from build123d import *

# Parameters (mm, degrees)
BOSS_EXTRUDE3_DEPTH = 25
SKETCH3_R           = 10
CUT_EXTRUDE1_DEPTH  = 25
SKETCH4_R           = 12.5
CUT_EXTRUDE2_DEPTH  = 15
SKETCH5_R           = 50
BOSS_EXTRUDE5_DEPTH = 75
SKETCH9_R           = 42.5
CUT_EXTRUDE5_DEPTH  = 15
SKETCH10_R          = 37.5
CUT_EXTRUDE6_DEPTH  = 60


with BuildPart() as part:
    # Sketch2 → Boss-Extrude3 (new body)
    with BuildSketch(Plane(origin=(0, 0, 0), x_dir=(1, 0, 0), z_dir=(0, 1, 0))):
        with BuildLine():
            Line((-125, 19.364916731), (-12.5, 48.412291828))
            ThreePointArc((-12.5, 48.412291828), (0, 50), (12.5, 48.412291828))
            Line((12.5, 48.412291828), (125, 19.364916731))
            ThreePointArc((125, 19.364916731), (140, 0), (125, -19.364916731))
            Line((125, -19.364916731), (12.5, -48.412291828))
            ThreePointArc((12.5, -48.412291828), (0, -50), (-12.5, -48.412291828))
            Line((-12.5, -48.412291828), (-125, -19.364916731))
            ThreePointArc((-125, -19.364916731), (-140, 0), (-125, 19.364916731))
        make_face()
    extrude(amount=BOSS_EXTRUDE3_DEPTH)

    # Sketch3 → Cut-Extrude1 (cut)
    with BuildSketch(Plane(origin=(0, 25, 0), x_dir=(1, 0, 0), z_dir=(0, 1, 0))):
        with Locations((-120, 0)):
            Circle(SKETCH3_R)
        with Locations((120, 0)):
            Circle(SKETCH3_R)
    extrude(amount=-CUT_EXTRUDE1_DEPTH, mode=Mode.SUBTRACT)

    # Sketch4 → Cut-Extrude2 (cut)
    with BuildSketch(Plane(origin=(0, 25, 0), x_dir=(1, 0, 0), z_dir=(0, 1, 0))):
        with Locations((-120, 0)):
            Circle(SKETCH4_R)
        with Locations((120, 0)):
            Circle(SKETCH4_R)
    extrude(amount=-CUT_EXTRUDE2_DEPTH, mode=Mode.SUBTRACT)

    # Sketch5 → Boss-Extrude5 (add)
    with BuildSketch(Plane(origin=(0, 0, 0), x_dir=(1, 0, 0), z_dir=(0, 1, 0))):
        Circle(SKETCH5_R)
    extrude(amount=BOSS_EXTRUDE5_DEPTH)

    # Sketch9 → Cut-Extrude5 (cut)
    with BuildSketch(Plane(origin=(0, 75, 0), x_dir=(1, 0, 0), z_dir=(0, 1, 0))):
        Circle(SKETCH9_R)
    extrude(amount=-CUT_EXTRUDE5_DEPTH, mode=Mode.SUBTRACT)

    # Sketch10 → Cut-Extrude6 (cut)
    with BuildSketch(Plane(origin=(0, 60, 0), x_dir=(1, 0, 0), z_dir=(0, 1, 0))):
        Circle(SKETCH10_R)
    extrude(amount=-CUT_EXTRUDE6_DEPTH, mode=Mode.SUBTRACT)


solid = part.part
Can you work these out from the model? Positions are in its coordinate system, mm. A direction names the side the tool comes from. Round coordinates to 2 decimals unless told otherwise and drop trailing zeros. Order: outer loops, then holes, each group sorted by start corner. A loop starts at its lowest first (then second) coordinate and runs counter-clockwise, first axis right, second up. Notation, with made-up numbers: (82, 17.25) -> (140, 17.25) arc R13 cw to (140, 34.25) -> close; hole circle Ø6 at (-15.75, -0.5). An arc over 180 degrees is marked (long way). Write each question's results on one line, items separated by ' | '. Start each with the question number.
Item 1: If we section it at A-A, the plane z = 0: State how many separate pieces and enclosed holes the cut face has, then the cut area to 4 significant figures.
Item 2: If we section it at B-B, the plane y = 5.5: Write out the boundary of the cut face in (x, z), then the cut area to 3 significant figures.
Item 3: If we section it at C-C, the plane x = 0: Write out the boundary of the cut face in (y, z), then the cut area to 4 significant figures.
Item 4: If we section it at D-D, the plane z = -33: Write out the boundary of the cut face in (x, y), then the cut area to 3 significant figures.
Item 5: Please list where these lines run through material, in increasing order: L1, parallel to X at y = 27, z = 0; L2, parallel to Y at x = 84, z = -22.5.
Item 6: Thinking about a two-plate mould opening in X: for faces 3 (the flat face through (77, 25, -1)), 4 (the cylindrical face through (131.923, 17.605, -3.755)), 5 (the flat face through (-69.538, 12.325, -33.685)), which applies, +X half, -X half, draft (parallel to the pull), parting line (faces both ways), or undercut?
Item 7: Will these pins go through, and if not, where does the flat tip stop? pin 1 (4 mm diameter, centred on x = -33.5, y = 20, fed in from +Z); pin 2 (1 mm diameter, centred on x = 21, y = 54.5, fed in from -Z); pin 3 (7.5 mm diameter, centred on x = -114, z = 2.5, fed in from +Y); pin 4 (18 mm diameter, centred on x = -120, z = 0, fed in from +Y).
Item 8: Which directions (+Z, -Z, +X, -X, +Y, -Y) give clear straight access to the entire face, cutting with the end or side of a thin tool? Please do faces 1 (the cylindrical face through (140, 12, 0)), 2 (the flat face through (119.9, 10, -10.2)).
Results:
1) separate pieces: 4 | enclosed holes: 0 | area: 5,075 mm2
2) outline: (-125, -19.36) -> (-12.5, -48.41) arc R50 ccw to (12.5, -48.41) -> (125, -19.36) arc R20 ccw to (125, 19.36) -> (12.5, 48.41) arc R50 ccw to (-12.5, 48.41) -> (-125, 19.36) arc R20 ccw to start; hole circle Ø20 at (-120, 0); hole circle Ø75 at (0, 0); hole circle Ø20 at (120, 0) | area: 13,500 mm2
3) outline: (0, -50) -> (75, -50) -> (75, -42.5) -> (60, -42.5) -> (60, -37.5) -> (0, -37.5) -> close; (0, 37.5) -> (60, 37.5) -> (60, 42.5) -> (75, 42.5) -> (75, 50) -> (0, 50) -> close | area: 1,725 mm2
4) outline: (-72.19, 0) -> (-17.81, 0) -> (-17.81, 60) -> (-26.78, 60) -> (-26.78, 75) -> (-37.56, 75) -> (-37.56, 25) -> (-72.19, 25) -> close; (17.81, 0) -> (72.19, 0) -> (72.19, 25) -> (37.56, 25) -> (37.56, 75) -> (26.78, 75) -> (26.78, 60) -> (17.81, 60) -> close | area: 4,430 mm2
5) L1: x = -50 to -37.5, 37.5 to 50 | L2: y = 0 to 25
6) face 3: draft | face 4: undercut | face 5: -X half
7) pin 1: stops at z = 43.51 | pin 2: stops at z = -45.6 | pin 3: stops at y = 10 | pin 4: passes through
8) face 1: +X, +Y, -Y | face 2: +Y
